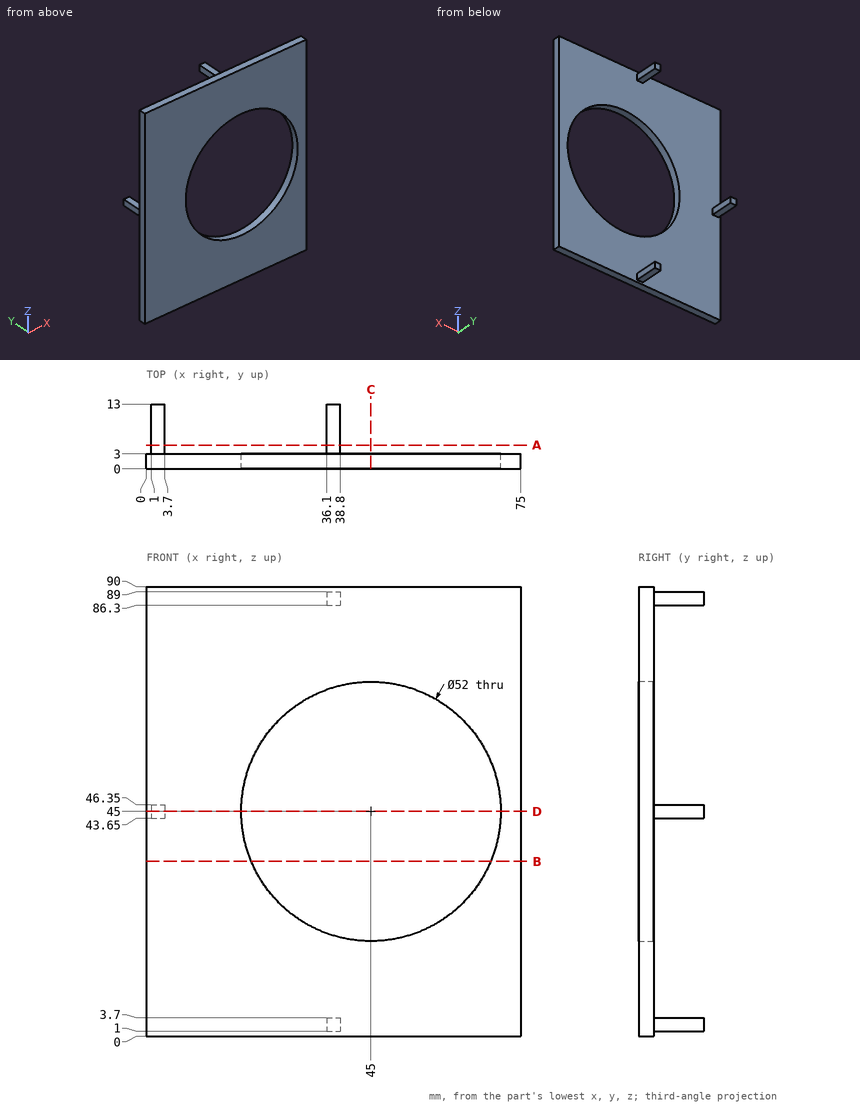
Geometry: see drawing. Coordinates: mm, zero at the bounding-box minimum. Give positions to 0.01 mm unless a question says otherwise; leave off trailing zeros. Order: outer loops, then holes, each group sorted by start corner. A loop starts at its lowest first (then second) coordinate and runs counter-clockwise, first axis right, second up.
1. Line query: probe 1 along X at (y, z) = (2.3, 45); probe 2 along Y at (x, z) = (10.5, 82); probe 3 along Z at (x, y) = (36, 1.5). Output: solid intervals per line, ascending.
Computed:
probe 1: x = 0 to 19, 71 to 75
probe 2: y = 0 to 3
probe 3: z = 0 to 20.61, 69.39 to 90
2. Cut plane A-A (y = 4.75). Return loops of the section in (x, z).
Computed:
outline: (1, 43.65) - (3.7, 43.65) - (3.7, 46.35) - (1, 46.35) - close; (36.1, 1) - (38.8, 1) - (38.8, 3.7) - (36.1, 3.7) - close; (36.1, 86.3) - (38.8, 86.3) - (38.8, 89) - (36.1, 89) - close
3. Cut plane B-B (z = 35). Return loops of the section in (x, y).
Computed:
outline: (0, 0) - (21, 0) - (21, 3) - (0, 3) - close; (69, 0) - (75, 0) - (75, 3) - (69, 3) - close
4. Cut plane C-C (x = 45). Return loops of the section in (y, z), and give its area (3 significant figures).
Computed:
outline: (0, 0) - (3, 0) - (3, 19) - (0, 19) - close; (0, 71) - (3, 71) - (3, 90) - (0, 90) - close
area: 114 mm2
5. Cut plane D-D (z = 45). Return loops of the section in (x, y), and give its area (3 significant figures).
Computed:
outline: (0, 0) - (19, 0) - (19, 3) - (3.7, 3) - (3.7, 13) - (1, 13) - (1, 3) - (0, 3) - close; (71, 0) - (75, 0) - (75, 3) - (71, 3) - close
area: 96.0 mm2
6. Pin query (flat end, axial travel): pin 1 Ø1 at (x, z) = (62, 15) entering from +Y; pin 2 Ø3 at (x, y) = (38, 9) entering from -Z; pin 3 Ø2 at (y, z) = (6.5, 45) entering from -X. Return the tip coordinate at first contact, or that it passes through.
Computed:
pin 1: stops at y = 3
pin 2: stops at z = 1
pin 3: stops at x = 1
